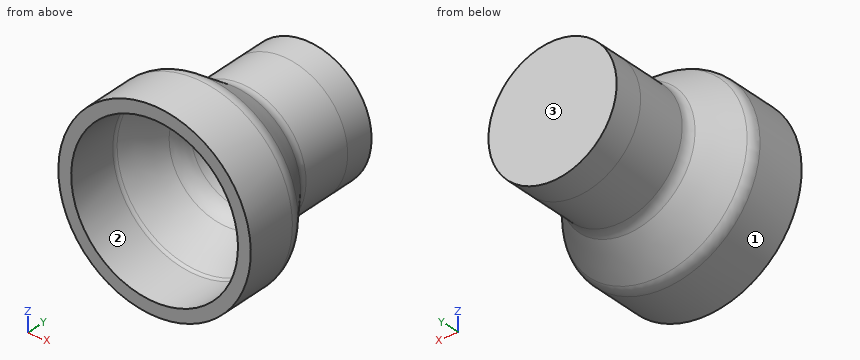
```python
from build123d import *

# Parameters (mm, degrees)
SKETCH8_R           = 2.5
BOSS_EXTRUDE1_DEPTH = 1.15


with BuildPart() as part:
    # Sketch6 → Revolve-Thin2 (revolve)
    with BuildSketch(Plane(origin=(0, 0, 0), x_dir=(0, 0, -1), z_dir=(1, 0, 0))):
        with BuildLine():
            Line((-3.75, 0), (-3.75, 2))
            ThreePointArc((-3.75, 2), (-3.712963507, 2.232772503), (-3.605511899, 2.442555466))
            Line((-3.605511899, 2.442555466), (-2.644488101, 3.757444534))
            ThreePointArc((-2.644488101, 3.757444534), (-2.537036493, 3.967227497), (-2.5, 4.2))
            Line((-2.5, 4.2), (-2.5, 6.2))
            Line((-2.5, 6.2), (-2, 6.2))
            Line((-2, 6.2), (-2, 4.2))
            ThreePointArc((-2, 4.2), (-2.061727489, 3.812045829), (-2.240813502, 3.462407557))
            Line((-2.240813502, 3.462407557), (-3.2018373, 2.147518489))
            ThreePointArc((-3.2018373, 2.147518489), (-3.237654502, 2.077590834), (-3.25, 2))
            Line((-3.25, 2), (-3.25, 0))
            Line((-3.25, 0), (-3.75, 0))
        make_face()
    revolve(axis=Axis((0, -0.227579974, 0), (0, 1, 0)))

    # Sketch8 → Boss-Extrude1 (add)
    with BuildSketch(Plane(origin=(0, 6.2, 0), x_dir=(1, 0, 0), z_dir=(0, 1, 0))):
        Circle(SKETCH8_R)
    extrude(amount=BOSS_EXTRUDE1_DEPTH)


solid = part.part
```
The listing builds one solid part. Answer for the finished solid, in the listing's coordinates (mm). Face numbers are marked on the shaded views. Give positions to 0.01 mm unless a question says otherwise; leave off trailing zeros. Order: outer loops, then holes, each group sorted by start corner. A loop starts at its lowest first (then second) coordinate and runs counter-clockwise, first axis right, second up. Notation, with made-up numbers: (57, 55.25) - (61, 55.25) arc R31 ccw to (61, 80.25) - close; hole circle Ø11 at (50.25, -18.75). An arc over 180 degrees is marked (long way). Use one line per item in the form item = value. Start each with the question number.
(1) Consider line 1 (X direction, y = 0.7, z = 0); line 2 (X direction, y = 4.7, z = 0); line 3 (Y direction, x = 0.5, z = -1.75). Determine where each line is inside the solid, lowest interval first. Write a range as from..to.
(2) A cutting plane is placed at A-A, the plane z = 0. Write down the section's boundary in (x, y), then the cut area to 3 significant figures.
(3) The mould has two halves that part along Z. Classify the marked faces 1, 2 and 3: released by +Z, released by -Z, zero draft, split by the parting line, or undercut.
(4) A cutting plane is placed at B-B, the plane y = 1.5. Write down the section's boundary in (x, z), then the cut area to 3 significant figures.
(5) Flat-ended cylindrical pins translate along their axes: pin 1 Ø1.2 at (x, z) = (0, 0.5) entering from -Y; pin 2 Ø1.5 at (x, y) = (0.5, 6) entering from +Z. Find the tip coordinate at first contact, or state that the pin passes through.
(6) A cutting plane is placed at D-D, the plane y = 6.75. Write down the section's boundary in (x, z).
(7) A cutting plane is placed at C-C, the plane x = 0. Write down the section's boundary in (y, z).
Ans:
q1.line_1 = -3.75..-3.25, 3.25..3.75
q1.line_2 = -2.5..-2, 2..2.5
q1.line_3 = 6.2..7.35
q2.outline = (-3.75, 0) - (-3.25, 0) - (-3.25, 2) arc R0.25 cw to (-3.2, 2.15) - (-2.24, 3.46) arc R1.25 ccw to (-2, 4.2) - (-2, 6.2) - (2, 6.2) - (2, 4.2) arc R1.25 ccw to (2.24, 3.46) - (3.2, 2.15) arc R0.25 cw to (3.25, 2) - (3.25, 0) - (3.75, 0) - (3.75, 2) arc R0.75 ccw to (3.61, 2.44) - (2.64, 3.76) arc R0.75 cw to (2.5, 4.2) - (2.5, 7.35) - (-2.5, 7.35) - (-2.5, 4.2) arc R0.75 cw to (-2.64, 3.76) - (-3.61, 2.44) arc R0.75 ccw to (-3.75, 2) - close
q2.area = 12.3 mm^2
q3.face_1 = split by the parting line
q3.face_2 = undercut
q3.face_3 = zero draft
q4.outline = circle Ø7.5 at (0, 0); hole circle Ø6.5 at (0, 0)
q4.area = 11.0 mm^2
q5.pin_1 = 6.2
q5.pin_2 = 2.5
q6.outline = circle Ø5 at (0, 0)
q7.outline = (0, -3.75) - (2, -3.75) arc R0.75 ccw to (2.44, -3.61) - (3.76, -2.64) arc R0.75 cw to (4.2, -2.5) - (7.35, -2.5) - (7.35, 2.5) - (4.2, 2.5) arc R0.75 cw to (3.76, 2.64) - (2.44, 3.61) arc R0.75 ccw to (2, 3.75) - (0, 3.75) - (0, 3.25) - (2, 3.25) arc R0.25 cw to (2.15, 3.2) - (3.46, 2.24) arc R1.25 ccw to (4.2, 2) - (6.2, 2) - (6.2, -2) - (4.2, -2) arc R1.25 ccw to (3.46, -2.24) - (2.15, -3.2) arc R0.25 cw to (2, -3.25) - (0, -3.25) - close
